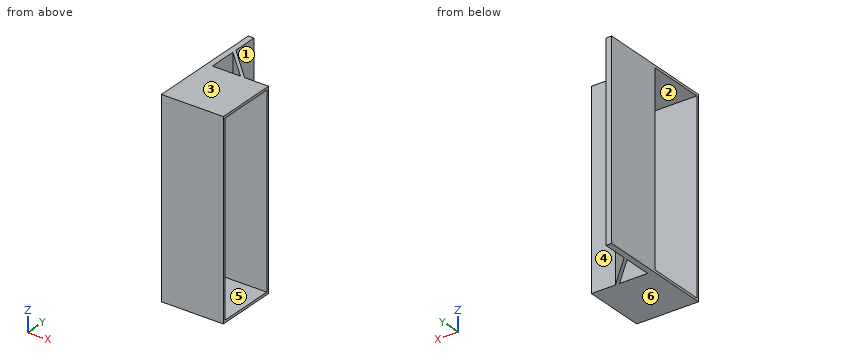
```python
from build123d import *

# Parameters (mm, degrees)
SKETCH_1_W          = 76
SKETCH_1_H          = 76
EXTRUDE_1_DEPTH     = 236
SKETCH_3_W          = 230
SKETCH_3_H          = 70
CUT_EXTRUDE_1_DEPTH = 130.085755737
SKETCH_4_W          = 7
SKETCH_4_H          = 236
EXTRUDE_2_DEPTH     = 70
EXTRUDE_5_DEPTH     = 236


with BuildPart() as part:
    # 草圖1 → 填料-伸長1 (new body)
    with BuildSketch(Plane.XY):
        with Locations((-8.891608392, -8.891608392)):
            Rectangle(SKETCH_1_W, SKETCH_1_H)
    extrude(amount=EXTRUDE_1_DEPTH)

    # 草圖3 → 除料-伸長1 (cut)
    with BuildSketch(Plane.ZY.offset(46.891608392)):
        with Locations((118, -8.891608392)):
            Rectangle(SKETCH_3_W, SKETCH_3_H)
    extrude(amount=-CUT_EXTRUDE_1_DEPTH, mode=Mode.SUBTRACT)

    # 草圖4 → 填料-伸長2 (add)
    with BuildSketch(Plane(origin=(0, 29.108391608, 0), x_dir=(1, 0, 0), z_dir=(0, 1, 0))):
        with Locations((-43.391608392, -118)):
            Rectangle(SKETCH_4_W, SKETCH_4_H)
    extrude(amount=EXTRUDE_2_DEPTH)

    # 草圖5 → 填料-伸長5 (add)
    with BuildSketch(Plane.XY.offset(236)):
        Polygon((-39.891608392, 63.608391608), (-5.391608392, 29.108391608), (-0.391608392, 29.108391608), (-39.891608392, 68.608391608), align=None)
    extrude(amount=-EXTRUDE_5_DEPTH)


solid = part.part
```
Source: CAD feature listing. Evaluate the final solid. Frame: model axes, mm. Face numbers are marked on the shaded views. A direction names the side the tool comes from. Coordinates: 2 decimals unless noted, no trailing zeros. Loops run counter-clockwise (first coordinate to the right, second up) from the corner with the lowest first, then second, coordinate; pieces in that order, holes last. Notation, with made-up numbers: M 68.25,-6 L 120.25,-6 A30 cw 120.25,16 Z; hole C 69.5,-36.75 d4. An arc over 180 degrees is marked long. Use a Markdown table: item, result. Add a question column.
Q1. Section query D-D, the plane x = 9. Return loops of the section in (y, z), and give its area (3 significant figures).
Q2. Section query B-B, the plane x = -8.5. Return loops of the section in (y, z), and give its area (3 significant figures).
Q3. Material intervals for L1, parallel to Y at x = 1.5, z = 182; L2, parallel to Y at x = -30, z = 37.5; L3, parallel to Y at x = -26, z = 183.5, sorted ascending.
Q4. First-contact query: pin 1 (9 mm diameter, centred on y = 85.5, z = 114, fed in from +X); pin 2 (4 mm diameter, centred on x = -32.5, z = 86.5, fed in from +Y); pin 3 (6 mm diameter, centred on x = -30.5, z = 109.5, fed in from +Y); pin 4 (21 mm diameter, centred on x = -26.5, y = -26, fed in from -Z). Flat tips, straight axial feed; report the tip coordinate or a pass-through.
Q5. Draft query along Y for the marked faces 4, 5 and 6. Return one class per face: pulls with the +Y half, pulls with the -Y half, needs draft (parallel to the pull), parting line crosses it, or undercut.
Q6. Access query for the marked faces 1, 2 and 3. Directions: +Z, -Z, +X, -X, +Y, -Y. A direction counts if a zero-diameter tool reaches every point of the face in a straight line with its end or side. Return the directions, or none.
Q7. Section query A-A, the plane z = 64.5. Return loops of the section in (x, y).
Q8. Section query C-C, the plane y = -28. Return loops of the section in (x, z), and give its area (3 significant figures).
Result:
| question | item | result |
|---|---|---|
| 1 | outline | M -46.89,0 L 29.11,0 L 29.11,236 L -46.89,236 Z; hole M -43.89,3 L 26.11,3 L 26.11,233 L -43.89,233 Z |
| 1 | area | 1,840 mm2 |
| 2 | outline | M -46.89,0 L 29.11,0 L 29.11,236 L -46.89,236 Z; M 32.22,0 L 37.22,0 L 37.22,236 L 32.22,236 Z; hole M -43.89,3 L 26.11,3 L 26.11,233 L -43.89,233 Z |
| 2 | area | 3,020 mm2 |
| 3 | L1 | y = -46.89 to -43.89, 26.11 to 29.11 |
| 3 | L2 | y = -46.89 to -43.89, 26.11 to 29.11, 53.72 to 58.72 |
| 3 | L3 | y = -46.89 to -43.89, 26.11 to 29.11, 49.72 to 54.72 |
| 4 | pin 1 | stops at x = -39.89 |
| 4 | pin 2 | stops at y = 63.22 |
| 4 | pin 3 | stops at y = 62.22 |
| 4 | pin 4 | stops at z = 0 |
| 5 | face 4 | pulls with the +Y half |
| 5 | face 5 | undercut |
| 5 | face 6 | needs draft |
| 6 | face 1 | +Z, -Z, +X, +Y |
| 6 | face 2 | +X, -X |
| 6 | face 3 | +Z, +X, -X, +Y, -Y |
| 7 | outline | M -46.89,-46.89 L 29.11,-46.89 L 29.11,-43.89 L -46.89,-43.89 Z; M -46.89,26.11 L 29.11,26.11 L 29.11,29.11 L -0.39,29.11 L -39.89,68.61 L -39.89,99.11 L -46.89,99.11 Z; hole M -39.89,29.11 L -5.39,29.11 L -39.89,63.61 Z |
| 8 | outline | M -46.89,0 L 29.11,0 L 29.11,3 L -46.89,3 Z; M -46.89,233 L 29.11,233 L 29.11,236 L -46.89,236 Z |
| 8 | area | 456 mm2 |
